from build123d import *

# Parameters (mm, degrees)
SKETCH1_W           = 96
SKETCH1_H           = 220
BOSS_EXTRUDE1_DEPTH = 25
CUT_EXTRUDE1_DEPTH  = 23.5
CUT_EXTRUDE2_REACH  = 248.327
CUT_EXTRUDE3_REACH  = 247.79
SKETCH4_R           = 1.75
SKETCH5_R           = 3
CUT_EXTRUDE4_DEPTH  = 5


with BuildPart() as part:
    # Sketch1 → Boss-Extrude1 (new body)
    with BuildSketch(Plane(origin=(0, 0, 0), x_dir=(1, 0, 0), z_dir=(0, 1, 0))):
        with Locations((48, 115.467836257)):
            Rectangle(SKETCH1_W, SKETCH1_H)
    extrude(amount=BOSS_EXTRUDE1_DEPTH)

    # Sketch2 → Cut-Extrude1 (cut)
    with BuildSketch(Plane(origin=(0, 25, 0), x_dir=(1, 0, 0), z_dir=(0, 1, 0))):
        with BuildLine():
            Line((2, 223.467836257), (2, 219.467836257))
            Line((2, 219.467836257), (6.5, 219.467836257))
            ThreePointArc((6.5, 219.467836257), (11, 214.967836257), (6.5, 210.467836257))
            Line((6.5, 210.467836257), (2, 210.467836257))
            Line((2, 210.467836257), (2, 39.467836257))
            Line((2, 39.467836257), (6.5, 39.467836257))
            ThreePointArc((6.5, 39.467836257), (11, 34.967836257), (6.5, 30.467836257))
            Line((6.5, 30.467836257), (2, 30.467836257))
            Line((2, 30.467836257), (2, 7.467836257))
            Line((2, 7.467836257), (94, 7.467836257))
            Line((94, 7.467836257), (94, 30.467836257))
            Line((94, 30.467836257), (89.5, 30.467836257))
            ThreePointArc((89.5, 30.467836257), (85, 34.967836257), (89.5, 39.467836257))
            Line((89.5, 39.467836257), (94, 39.467836257))
            Line((94, 39.467836257), (94, 210.467836257))
            Line((94, 210.467836257), (89.5, 210.467836257))
            ThreePointArc((89.5, 210.467836257), (85, 214.967836257), (89.5, 219.467836257))
            Line((89.5, 219.467836257), (94, 219.467836257))
            Line((94, 219.467836257), (94, 223.467836257))
            Line((94, 223.467836257), (2, 223.467836257))
        make_face()
    extrude(amount=-CUT_EXTRUDE1_DEPTH, mode=Mode.SUBTRACT)

    # Cut-Extrude2: up to this face of the body (flat: up to its plane)
    cut_extrude2_end = Plane(part.part.faces().sort_by_distance((0, 12.5, -115.467836257))[0])
    # Sketch3 → Cut-Extrude2 (cut, up to the picked face)
    with BuildSketch(Plane(origin=(96, 0, 0), x_dir=(0, 0, -1), z_dir=(1, 0, 0)), mode=Mode.PRIVATE) as cut_extrude2_sk1:
        with BuildLine():
            Line((225.467836257, 6), (29.467836257, 6))
            ThreePointArc((29.467836257, 6), (22.396768445, 8.928932188), (19.467836257, 16))
            Line((19.467836257, 16), (19.467836257, 25))
            Line((19.467836257, 25), (225.467836257, 25))
            Line((225.467836257, 25), (225.467836257, 6))
        make_face()
    cut_extrude2_tool1 = split(extrude(cut_extrude2_sk1.sketch, amount=-CUT_EXTRUDE2_REACH, mode=Mode.PRIVATE), bisect_by=cut_extrude2_end, keep=Keep.BOTH, mode=Mode.PRIVATE)
    add(cut_extrude2_tool1.solids().sort_by(Axis((96, 15.54006, -123.023377), (-1, 0, 0)))[0], mode=Mode.SUBTRACT)

    # Sketch4 → Cut-Extrude3 (cut, up to next)
    with BuildSketch(Plane(origin=(0, 6, 0), x_dir=(1, 0, 0), z_dir=(0, 1, 0)), mode=Mode.PRIVATE) as cut_extrude3_sk1:
        with Locations(Location((6.5, 34.967836257, 0), (0, 0, 270))):
            Circle(SKETCH4_R)
    cut_extrude3_tool1 = extrude(cut_extrude3_sk1.sketch, amount=-CUT_EXTRUDE3_REACH, mode=Mode.PRIVATE) & part.part
    # Sketch4 → Cut-Extrude3 (cut, up to next)
    with BuildSketch(Plane(origin=(0, 6, 0), x_dir=(1, 0, 0), z_dir=(0, 1, 0)), mode=Mode.PRIVATE) as cut_extrude3_sk2:
        with Locations(Location((89.5, 34.967836257, 0), (0, 0, 270))):
            Circle(SKETCH4_R)
    cut_extrude3_tool2 = extrude(cut_extrude3_sk2.sketch, amount=-CUT_EXTRUDE3_REACH, mode=Mode.PRIVATE) & part.part
    # Sketch4 → Cut-Extrude3 (cut, up to next)
    with BuildSketch(Plane(origin=(0, 6, 0), x_dir=(1, 0, 0), z_dir=(0, 1, 0)), mode=Mode.PRIVATE) as cut_extrude3_sk3:
        with Locations(Location((89.5, 214.967836257, 0), (0, 0, 270))):
            Circle(SKETCH4_R)
    cut_extrude3_tool3 = extrude(cut_extrude3_sk3.sketch, amount=-CUT_EXTRUDE3_REACH, mode=Mode.PRIVATE) & part.part
    # Sketch4 → Cut-Extrude3 (cut, up to next)
    with BuildSketch(Plane(origin=(0, 6, 0), x_dir=(1, 0, 0), z_dir=(0, 1, 0)), mode=Mode.PRIVATE) as cut_extrude3_sk4:
        with Locations(Location((6.5, 214.967836257, 0), (0, 0, 270))):
            Circle(SKETCH4_R)
    cut_extrude3_tool4 = extrude(cut_extrude3_sk4.sketch, amount=-CUT_EXTRUDE3_REACH, mode=Mode.PRIVATE) & part.part
    add(cut_extrude3_tool1.solids().sort_by_distance((6.5, 6, -34.967836))[0], mode=Mode.SUBTRACT)
    add(cut_extrude3_tool2.solids().sort_by_distance((89.5, 6, -34.967836))[0], mode=Mode.SUBTRACT)
    add(cut_extrude3_tool3.solids().sort_by_distance((89.5, 6, -214.967836))[0], mode=Mode.SUBTRACT)
    add(cut_extrude3_tool4.solids().sort_by_distance((6.5, 6, -214.967836))[0], mode=Mode.SUBTRACT)

    # Sketch5 → Cut-Extrude4 (cut)
    with BuildSketch(Plane.XZ):
        with Locations(Location((6.5, -34.967836257, 0), (0, 0, 270))):
            Circle(SKETCH5_R)
        with Locations(Location((89.5, -34.967836257, 0), (0, 0, 270))):
            Circle(SKETCH5_R)
        with Locations(Location((6.5, -214.967836257, 0), (0, 0, 270))):
            Circle(SKETCH5_R)
        with Locations((98.5, -214.967836257)):
            Circle(SKETCH5_R)
    extrude(amount=-CUT_EXTRUDE4_DEPTH, mode=Mode.SUBTRACT)


solid = part.part
Can you work these out from the model? Positions are in its coordinate system, mm. A direction names the side the tool comes from. Round coordinates to 2 decimals unless told otherwise and drop trailing zeros. Loops run counter-clockwise (first coordinate to the right, second up) from the corner with the lowest first, then second, coordinate; pieces in that order, holes last. Notation, with made-up numbers: (27.25, 5.5) - (51.25, 5.5) arc R21 cw to (51.25, 30.5) - close; hole circle Ø9 at (87.5, 14.25). An arc over 180 degrees is marked (long way). Answer in a Markdown table with one row per item. Add a question column.
Q1. For pin 1 Ø0.6 at (x, y) = (95, 21) entering from -Z; pin 2 Ø12 at (y, z) = (5.5, -44.5) entering from -X; pin 3 Ø12 at (x, z) = (17, -94) entering from +Y; pin 4 Ø5.5 at (x, z) = (6.5, -34.97) entering from +Y, each with a flat end and sliding along its axis, tell me the tip position at first contact or that it passes through.
Q2. I need wall thicknesses on L1, parallel to Z at x = 89.5, y = 5.85; L2, parallel to Z at x = 86, y = 4; L3, parallel to X at y = 1.75, z = -176.5. Which ranges of each line are inside material? Lowest first, please.
Q3. I want a section at A-A on z = -106. List the corners of the cut face in (x, y) for me, and give its area (3 significant figures).
Q4. Which directions (+Z, -Z, +X, -X, +Y, -Y) give clear straight access to the entire face, cutting with the end or side of a thin tool? Please do faces 4 (the flat face through (87.5, 5, -34.9)), 5 (the cylindrical face through (11, 4, -35)), 6 (the flat face through (47, 3, -225.468)).
Q5. We'd pull the mould along X, two halves only. Please class faces 1 (the flat face through (0, 4, -99)), 2 (the flat face through (49, 4, -223.468)), 3 (the flat face through (41, 25, -7)): pulls with the +X half, pulls with the -X half, needs draft (parallel to the pull), parting line crosses it, or undercut.
Q6. I want a section at B-B on x = 24. List the corners of the cut face in (y, z) for me, and give its area (3 significant figures).
A:
| question | item | result |
|---|---|---|
| 1 | pin 1 | z = -19.47 |
| 1 | pin 2 | x = 0 |
| 1 | pin 3 | y = 1.5 |
| 1 | pin 4 | y = 6 |
| 2 | L1 | -225.47 to -223.47, -219.47 to -216.72, -213.22 to -210.47, -39.47 to -36.72, -33.22 to -30.47, -7.47 to -5.47 |
| 2 | L2 | -225.47 to -223.47, -217.8 to -212.14, -37.8 to -32.14, -7.47 to -5.47 |
| 2 | L3 | 0 to 2, 94 to 96 |
| 3 | outline | (0, 0) - (96, 0) - (96, 6) - (94, 6) - (94, 1.5) - (2, 1.5) - (2, 6) - (0, 6) - close |
| 3 | area | 162 mm^2 |
| 4 | face 4 | -Y |
| 4 | face 5 | +Y |
| 4 | face 6 | -Z, +X, -X, +Y, -Y |
| 5 | face 1 | pulls with the -X half |
| 5 | face 2 | undercut |
| 5 | face 3 | needs draft |
| 6 | outline | (0, -225.47) - (6, -225.47) - (6, -223.47) - (1.5, -223.47) - (1.5, -7.47) - (25, -7.47) - (25, -5.47) - (0, -5.47) - close |
| 6 | area | 386 mm^2 |
